```python
from build123d import *

# Parameters (mm, degrees)
F0_W     = 106.68
F0_H     = 17.78
F1_DEPTH = 2.54
F2_R     = 2.54
F3_W     = 81.28
F3_H     = 1.27
F4_DEPTH = 25.4
F5_W     = 81.28
F5_H     = 15.24
F6_DEPTH = 0.508
F7_W     = 81.28
F7_H     = 16.51
F8_DEPTH = 0.508


with BuildPart() as f1:
    # F0 (on Top) → F1 (new body)
    with BuildSketch(Plane.XY):
        with Locations((53.34, 8.89)):
            Rectangle(F0_W, F0_H)
    extrude(amount=F1_DEPTH)

    # F2
    f2_edges = [f1.edges().sort_by_distance(p)[0] for p in [
        (106.68, 17.78, 1.27),
        (106.68, 0, 1.27),
        (0, 17.78, 1.27),
        (0, 0, 1.27),
    ]]
    fillet(f2_edges, radius=F2_R)

    # F3 (on face) → F4 (cut)
    with BuildSketch(Plane.XY.offset(2.54)):
        with Locations((53.34, 17.145)):
            Rectangle(F3_W, F3_H)
        with Locations((53.34, 0.635)):
            Rectangle(F3_W, F3_H)
    extrude(amount=-F4_DEPTH, mode=Mode.SUBTRACT)

    # F5 (on face) → F6 (cut)
    with BuildSketch(Plane.XY.offset(2.54)):
        with Locations((53.34, 8.89)):
            Rectangle(F5_W, F5_H)
    extrude(amount=-F6_DEPTH, mode=Mode.SUBTRACT)

    # F7 (on face) → F8 (cut)
    with BuildSketch(Plane(origin=(0, 0, 0), x_dir=(1, 0, 0), z_dir=(0, 0, -1))):
        with Locations((53.34, -8.255)):
            Rectangle(F7_W, F7_H)
    extrude(amount=-F8_DEPTH, mode=Mode.SUBTRACT)


solid = f1.part
```
Build history of the part. All positions in model axes, mm. A direction names the side the tool comes from. Give positions to 0.01 mm unless a question says otherwise; leave off trailing zeros. Loops run counter-clockwise (first coordinate to the right, second up) from the corner with the lowest first, then second, coordinate; pieces in that order, holes last.
1) Probe line 1 along X through (y, z) = (12.75, 0.4); line 2 along Z through (x, y) = (18.5, 4); line 3 along Y through (x, z) = (32.5, 0.6). List the from-to ranges inside material, lowest first.
Values follow:
line 1: x = 0 to 12.7, 93.98 to 106.68
line 2: z = 0.51 to 2.03
line 3: y = 1.27 to 16.51
2) Band-saw the part on C-C on x = 80. List the corners of the cut face in (y, z).
Values follow:
outline: (1.27, 0.51) - (16.51, 0.51) - (16.51, 2.03) - (1.27, 2.03) - close
3) Drop flat-ended pins along their axis: P1, Ø4.5, axis at x = 36, y = 10.5, coming from the -Z side; P2, Ø2, axis at x = 65, y = 5.5, coming from the +Z side; P3, Ø0.5, axis at x = 65.5, z = 1.5, coming from the +Y side. Give the stop position or say it passes through.
Values follow:
P1: stops at z = 0.51
P2: stops at z = 2.03
P3: stops at y = 16.51
4) Two-plate mould, pull along X, no slides. Class faces 1 (the face through (8, 0, 1)), 2 (the face through (93.98, 8.8, 0.2)), 3 (the face through (53, 9, 0.508)), 4 (the face through (0.724, 17.016, 1.288)): released by +X, released by -X, zero draft, split by the parting line, or undercut.
Values follow:
face 1: zero draft
face 2: undercut
face 3: undercut
face 4: released by -X
5) Band-saw the part on B-B on z = 1.25. List the corners of the cut face in (x, y), then the cut area to 3 significant figures.
Values follow:
outline: (0, 2.54) arc R2.54 ccw to (2.54, 0) - (12.7, 0) - (12.7, 1.27) - (93.98, 1.27) - (93.98, 0) - (104.14, 0) arc R2.54 ccw to (106.68, 2.54) - (106.68, 15.24) arc R2.54 ccw to (104.14, 17.78) - (93.98, 17.78) - (93.98, 16.51) - (12.7, 16.51) - (12.7, 17.78) - (2.54, 17.78) arc R2.54 ccw to (0, 15.24) - close
area: 1,680 mm2
6) Band-saw the part on A-A on y = 5.5. List the corners of the cut face in (x, z).
Values follow:
outline: (0, 0) - (12.7, 0) - (12.7, 0.51) - (93.98, 0.51) - (93.98, 0) - (106.68, 0) - (106.68, 2.54) - (93.98, 2.54) - (93.98, 2.03) - (12.7, 2.03) - (12.7, 2.54) - (0, 2.54) - close
7) 3-axis set-ups, long thin cutter, end or side, ignore diameter. For faces 5 (the face through (53, 9, 2.032)), 6 (the face through (6, 9, 0)): which of +Z, -Z, +X, -X, +Y, -Y reach the whole face in a straight line?
Values follow:
face 5: +Z, +Y, -Y
face 6: -Z, +X, -X, +Y, -Y
